from build123d import *

# Parameters (mm, degrees)
SKETCH2_R           = 165
BOSS_EXTRUDE1_DEPTH = 13
SKETCH3_R           = 165
SKETCH3_R_2         = 149
CUT_EXTRUDE1_DEPTH  = 3
SKETCH4_R           = 152
CUT_EXTRUDE2_DEPTH  = 6
CUT_EXTRUDE3_DEPTH  = 5


with BuildPart() as part:
    # Sketch2 → Boss-Extrude1 (new body)
    with BuildSketch(Plane(origin=(0, 0, 0), x_dir=(1, 0, 0), z_dir=(0, 1, 0))):
        Circle(SKETCH2_R)
    extrude(amount=BOSS_EXTRUDE1_DEPTH)

    # Sketch3 → Cut-Extrude1 (cut)
    with BuildSketch(Plane.XZ):
        Circle(SKETCH3_R)
        Circle(SKETCH3_R_2, mode=Mode.SUBTRACT)
    extrude(amount=-CUT_EXTRUDE1_DEPTH, mode=Mode.SUBTRACT)

    # Sketch4 → Cut-Extrude2 (cut)
    with BuildSketch(Plane(origin=(0, 13, 0), x_dir=(1, 0, 0), z_dir=(0, 1, 0))):
        Circle(SKETCH4_R)
    extrude(amount=-CUT_EXTRUDE2_DEPTH, mode=Mode.SUBTRACT)

    # Sketch5 → Cut-Extrude3 (cut)
    with BuildSketch(Plane(origin=(0, 7, 0), x_dir=(1, 0, 0), z_dir=(0, 1, 0))):
        with BuildLine():
            Line((-4.5, -115.678465615), (-4.5, -22.794228634))
            ThreePointArc((-4.5, -22.794228634), (-7.794228634, -19.5), (-9, -15))
            Line((-9, -15), (-9, 15))
            ThreePointArc((-9, 15), (0, 24), (9, 15))
            Line((9, 15), (9, -15))
            ThreePointArc((9, -15), (7.794228634, -19.5), (4.5, -22.794228634))
            Line((4.5, -22.794228634), (4.5, -115.678465615))
            Line((4.5, -115.678465615), (20, -115.678465615))
            Line((20, -115.678465615), (20, -150.678465615))
            ThreePointArc((20, -150.678465615), (0, -152), (-20, -150.678465615))
            Line((-20, -150.678465615), (-20, -115.678465615))
            Line((-20, -115.678465615), (-4.5, -115.678465615))
        make_face()
    extrude(amount=-CUT_EXTRUDE3_DEPTH, mode=Mode.SUBTRACT)


solid = part.part
Read the model definition and answer for the solid it produces. Units are mm, in the model's axes. A direction names the side the tool comes from. Round coordinates to 2 decimals unless told otherwise and drop trailing zeros. Order: outer loops, then holes, each group sorted by start corner. A loop starts at its lowest first (then second) coordinate and runs counter-clockwise, first axis right, second up.
1) The part is cut by section B-B on z = 0. Write down the section's boundary in (x, y), plus the area to 3 significant figures.
2) The mould has two halves that part along Z. Classify faces 1 (the face through (-32.3, 1.479, -145.457)), 2 (the face through (0, 5, -24)), 3 (the face through (73, 13, 134)): released by +Z, released by -Z, zero draft, split by the parting line, or undercut.
3) Flat-ended cylindrical pins translate along their axes: pin 1 (5.5 mm diameter, centred on y = 3.5, z = 57.5, fed in from -X); pin 2 (4 mm diameter, centred on y = 4, z = 127.5, fed in from -X); pin 3 (1 mm diameter, centred on x = -84, y = 7.5, fed in from -Z). Find the tip coordinate at first contact, or state that the pin passes through.
4) The part is cut by section D-D on z = -102. Write down the section's boundary in (x, y), plus the area to 3 significant figures.
5) For faces 4 (the face through (32, 7, -3)), 5 (the face through (-35.769, 7.93, 161.076)), 6 (the face through (-25.2, 3, 147.4)), determine the directions among +Z, -Z, +X, -X, +Y, -Y from which every point of the face is accessible in a straight line to the end or side of a thin tool.
6) The part is cut by section C-C on x = -124.5. Write down the section's boundary in (y, z).
7) Straight lines are drawn through the part: L1, parallel to Z at x = 0, y = 9.95; L2, parallel to Z at x = -8, y = 5.5. For each, find the intervals that lie inside material, in ascending order.
8) The part is cut by section A-A on x = 0. Write down the section's boundary in (y, z).
Resolved:
1. outline: (-165, 3) - (-149, 3) - (-149, 0) - (149, 0) - (149, 3) - (165, 3) - (165, 13) - (152, 13) - (152, 7) - (9, 7) - (9, 2) - (-9, 2) - (-9, 7) - (-152, 7) - (-152, 13) - (-165, 13) - close
1. area: 2,280 mm2
2. face 1: split by the parting line
2. face 2: undercut
2. face 3: zero draft
3. pin 1: stops at x = -155.65
3. pin 2: stops at x = -107.12
3. pin 3: stops at z = -142.31
4. outline: (-129.7, 3) - (-108.61, 3) - (-108.61, 0) - (108.61, 0) - (108.61, 3) - (129.7, 3) - (129.7, 13) - (112.69, 13) - (112.69, 7) - (-112.69, 7) - (-112.69, 13) - (-129.7, 13) - close
4. area: 1,890 mm2
5. face 4: +Y
5. face 5: +Y, -Y
5. face 6: -Y
6. outline: (0, -81.86) - (3, -81.86) - (3, -108.28) - (13, -108.28) - (13, -87.2) - (7, -87.2) - (7, 87.2) - (13, 87.2) - (13, 108.28) - (3, 108.28) - (3, 81.86) - (0, 81.86) - close
7. L1: z = -165 to -152, 152 to 165
7. L2: z = -164.81 to -19.12, 19.12 to 115.68, 151.79 to 164.81
8. outline: (0, -149) - (3, -149) - (3, -165) - (13, -165) - (13, -152) - (7, -152) - (7, -24) - (2, -24) - (2, 149) - (0, 149) - close; (3, 152) - (13, 152) - (13, 165) - (3, 165) - close
